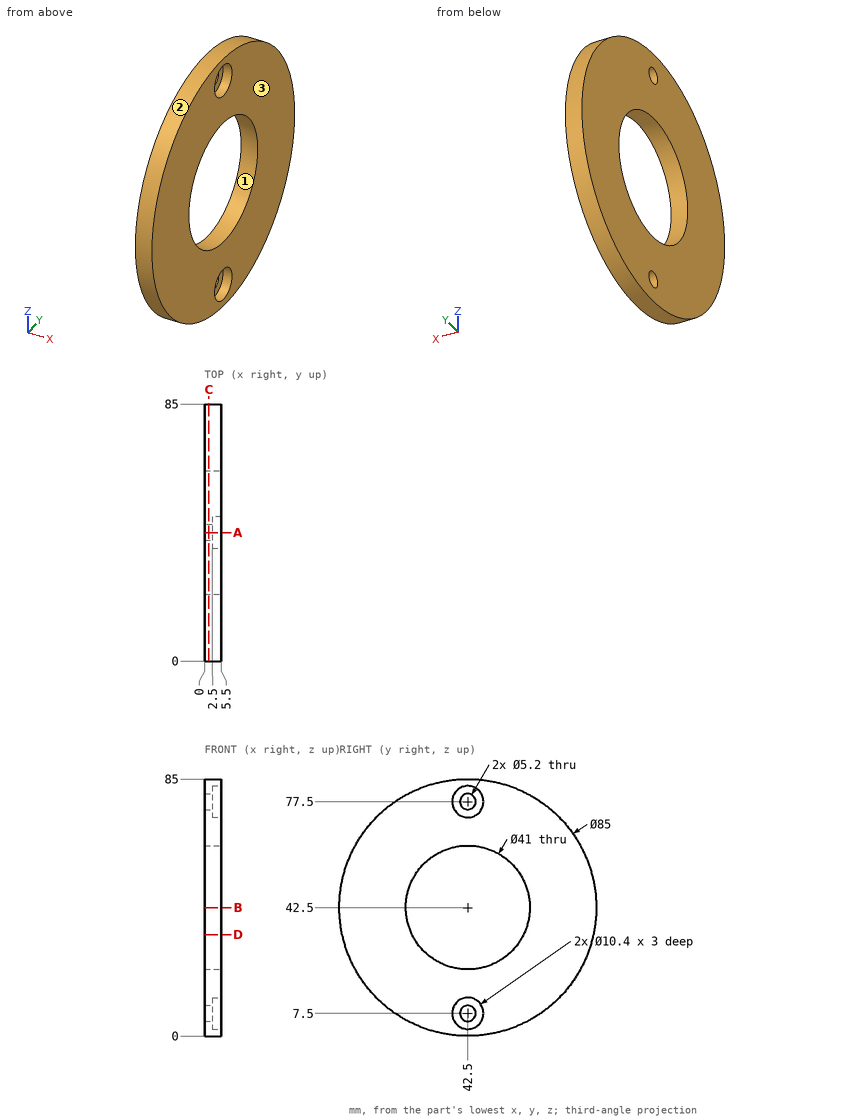
Job drawing, mm, ordinate dimensions from the low corner. One solid piece. Give positions to 0.01 mm unless a question says otherwise; leave off trailing zeros. Loops run counter-clockwise (first coordinate to the right, second up) from the corner with the lowest first, then second, coordinate; pieces in that order, holes last. Notation, with made-up numbers: (24, 32.25) -> (40, 32.25) arc R16 cw to (40, 50.25) -> close; hole circle Ø5 at (17, 4.5). An arc over 180 degrees is marked (long way). Write each question's results on one line, items separated by ' | '. Start each with the question number.
Q1. Band-saw the part on B-B on z = 42.5. List the corners of the cut face in (x, y).
Q2. Wall check: L1, parallel to Z at x = 2.25, y = 48; L2, parallel to Y at x = 1.95, z = 77.5; L3, parallel to Z at x = 1.85, y = 50. Give the ranges that are in metal, low to high.
Q3. Pin check, flat tips, straight feed: P1, Ø8.5, axis at y = 42.5, z = 78, coming from the +X side; P2, Ø2, axis at x = 2.5, y = 15, coming from the -Z side; P3, Ø2, axis at x = 5, z = 69.5, coming from the +Y side; P4, Ø4, axis at y = 42.5, z = 77.5, coming from the +X side. Stop position of each tip, or through.
Q4. Band-saw the part on D-D on z = 33.5. List the corners of the cut face in (x, y), plus the area to 3 significant figures.
Q5. Pull direction Y, two halves, no side cores. Call the marked faces 1, 2 and 3: +Y half, -Y half, draft (parallel to the pull), parting line (faces both ways), or undercut.
Q6. Band-saw the part on C-C on x = 1.35. List the corners of the cut face in (y, z), plus the area to 3 significant figures.
Q7. Band-saw the part on A-A on y = 42.5. List the corners of the cut face in (x, z), plus the area to 3 significant figures.
Results are:
1) outline: (0, 0) -> (5.5, 0) -> (5.5, 22) -> (0, 22) -> close; (0, 63) -> (5.5, 63) -> (5.5, 85) -> (0, 85) -> close
2) L1: z = 0.36 to 22.75, 62.25 to 84.64 | L2: y = 18.39 to 39.9, 45.1 to 66.61 | L3: z = 0.67 to 23.42, 61.58 to 84.33
3) P1: stops at x = 2.5 | P2: stops at z = 9.27 | P3: stops at y = 76.12 | P4: passes through
4) outline: (0, 0.96) -> (5.5, 0.96) -> (5.5, 24.08) -> (0, 24.08) -> close; (0, 60.92) -> (5.5, 60.92) -> (5.5, 84.04) -> (0, 84.04) -> close | area: 254 mm²
5) face 1: undercut | face 2: parting line | face 3: draft
6) outline: circle Ø85 at (42.5, 42.5); hole circle Ø41 at (42.5, 42.5); hole circle Ø5.2 at (42.5, 7.5); hole circle Ø5.2 at (42.5, 77.5) | area: 4,310 mm²
7) outline: (0, 0) -> (5.5, 0) -> (5.5, 2.3) -> (2.5, 2.3) -> (2.5, 4.9) -> (0, 4.9) -> close; (0, 10.1) -> (2.5, 10.1) -> (2.5, 12.7) -> (5.5, 12.7) -> (5.5, 22) -> (0, 22) -> close; (0, 63) -> (5.5, 63) -> (5.5, 72.3) -> (2.5, 72.3) -> (2.5, 74.9) -> (0, 74.9) -> close; (0, 80.1) -> (2.5, 80.1) -> (2.5, 82.7) -> (5.5, 82.7) -> (5.5, 85) -> (0, 85) -> close | area: 154 mm²
